Geometry: final body of the model. Coordinates: model frame, mm. A direction names the side the tool comes from. Round coordinates to 2 decimals unless told otherwise and drop trailing zeros. Write each loop counter-clockwise with the first axis right and the second up, starting at its lowest first coordinate (ties: lowest second). Pieces come first, ordered by that corner, then holes. Notation, with made-up numbers: (29, -38) -> (38, -38) arc R25 cw to (38, -14) -> close; hole circle Ø8 at (17.25, 13). An arc over 180 degrees is marked (long way). One line per item, written item: value. Start each with the question number.
from build123d import *

# Parameters (mm, degrees)
BOSS_EXTRUDE1_DEPTH            = 6.4
SKETCH2_R                      = 6.92820323
BOSS_EXTRUDE2_DEPTH            = 9.2
SKETCH3_R                      = 1.65
CUT_EXTRUDE3_DEPTH             = 16.6
SKETCH4_W                      = 5.65
SKETCH4_H                      = 2.55
CUT_EXTRUDE4_DEPTH             = 6.4
CUT_EXTRUDE5_REACH             = 4.978
SKETCH5_R                      = 1.5
CUT_EXTRUDE5_DIRECTION_2_REACH = 12.878
CUT_EXTRUDE7_DEPTH             = 2.55
SKETCH3_4_R                    = 2.05
SKETCH3_4_R_2                  = 1.65
CUT_EXTRUDE8_DEPTH             = 9.4
CHAMFER1_SIZE                  = 0.3


with BuildPart() as part:
    # Sketch1 → Boss-Extrude1 (new body)
    with BuildSketch(Plane(origin=(0, 0, 0), x_dir=(1, 0, 0), z_dir=(0, 1, 0))):
        Polygon((3.170646703, -6.160113594), (6.920138214, -0.334196206), (3.749491511, 5.825917388), (-3.170646703, 6.160113594), (-6.920138214, 0.334196206), (-3.749491511, -5.825917388), align=None)
    extrude(amount=BOSS_EXTRUDE1_DEPTH)

    # Sketch2 → Boss-Extrude2 (add)
    with BuildSketch(Plane(origin=(0, 6.4, 0), x_dir=(1, 0, 0), z_dir=(0, 1, 0))):
        Circle(SKETCH2_R)
    extrude(amount=BOSS_EXTRUDE2_DEPTH)

    # Sketch3 → Cut-Extrude3 (cut, through all)
    with BuildSketch(Plane(origin=(0, 15.6, 0), x_dir=(1, 0, 0), z_dir=(0, 1, 0))):
        Circle(SKETCH3_R)
    extrude(amount=-CUT_EXTRUDE3_DEPTH, mode=Mode.SUBTRACT)

    # Sketch4 → Cut-Extrude4 (cut)
    with BuildSketch(Plane(origin=(0, 15.6, 0), x_dir=(1, 0, 0), z_dir=(0, 1, 0))):
        with Locations((0, 2.675)):
            Rectangle(SKETCH4_W, SKETCH4_H)
    extrude(amount=-CUT_EXTRUDE4_DEPTH, mode=Mode.SUBTRACT)

    # Sketch5 → Cut-Extrude5 (cut, up to next)
    with BuildSketch(Plane.XY.offset(-3.95), mode=Mode.PRIVATE) as cut_extrude5_sk1:
        with Locations((0, 10.8)):
            Circle(SKETCH5_R)
    cut_extrude5_tool1 = extrude(cut_extrude5_sk1.sketch, amount=-CUT_EXTRUDE5_REACH, mode=Mode.PRIVATE) & part.part
    add(cut_extrude5_tool1.solids().sort_by_distance((0, 10.8, -3.95))[0], mode=Mode.SUBTRACT)

    # Sketch5 → Cut-Extrude5 direction 2 (cut, up to next)
    with BuildSketch(Plane.XY.offset(-3.95), mode=Mode.PRIVATE) as cut_extrude5_direction_2_sk1:
        with Locations((0, 10.8)):
            Circle(SKETCH5_R)
    cut_extrude5_direction_2_tool1 = extrude(cut_extrude5_direction_2_sk1.sketch, amount=CUT_EXTRUDE5_DIRECTION_2_REACH, mode=Mode.PRIVATE) & part.part
    add(cut_extrude5_direction_2_tool1.solids().sort_by_distance((0, 10.8, -3.95))[0], mode=Mode.SUBTRACT)

    # Sketch7 → Cut-Extrude7 (cut)
    with BuildSketch(Plane.XY.offset(-3.95)):
        Polygon((-2.825, 12.437789047), (-2.830866921, 9.172372758), (-0.005866921, 7.534583711), (2.825, 9.162210953), (2.830866921, 12.427627242), (0.005866921, 14.065416289), align=None)
    extrude(amount=CUT_EXTRUDE7_DEPTH, mode=Mode.SUBTRACT)

    # Sketch3_4 → Cut-Extrude8 (cut)
    with BuildSketch(Plane(origin=(0, 15.6, 0), x_dir=(1, 0, 0), z_dir=(0, 1, 0))):
        Circle(SKETCH3_4_R)
        Circle(SKETCH3_4_R_2, mode=Mode.SUBTRACT)
    extrude(amount=-CUT_EXTRUDE8_DEPTH, mode=Mode.SUBTRACT)

    # Chamfer1
    chamfer1_edges = [part.edges().sort_by_distance(p)[0] for p in [
        (-1.65, 0, 0),
        (-5.334814862, 0, 2.745860591),
        (-5.045392458, 0, -3.2471549),
        (0.289422404, 0, -5.993015491),
        (5.334814862, 0, -2.745860591),
        (5.045392458, 0, 3.2471549),
        (-0.289422404, 0, 5.993015491),
    ]]
    chamfer(chamfer1_edges, length=CHAMFER1_SIZE)


solid = part.part
(1) Set-up query: faces 5 (the face through (-5.3, 6.4, -3.5)), 6 (the face through (-1.438, 8.365, -2.693)), 7 (the face through (5.3, 6.4, 3.4)), 8 (the face through (-0.3, 6.4, 6.4)), 9 (the face through (0.34, 3.31, -5.99)). Return all of +Z, -Z, +X, -X, +Y, -Y with unobstructed straight access to the full face (end or side cutting, diameter ignored); none if empty.
(2) Line query: probe 1 along Y at (x, z) = (-5.25, 3); probe 2 along Y at (x, z) = (0, -4.55); probe 3 along X at (y, z) = (10.8, -6.25). Output: solid intervals per line, ascending.
(3) Pin query (flat end, axial travel): pin 1 (3.5 mm diameter, centred on x = 0, z = 0, fed in from -Y); pin 2 (3.5 mm diameter, centred on x = 0, z = 0, fed in from +Y); pin 3 (4 mm diameter, centred on x = 4.5, y = 4.5, fed in from +Z). Return the tip coordinate at first contact, or that it passes through.
(4) Section query D-D (x = -0.5). Count the separate pieces of the cut face and the enclosed holes in it, and give its area (3 significant figures).
(5) Section query A-A (y = 4.25). Output: boundary loops of the cut face in (x, z).
(6) Pull-direction query (X, two-part tool) for faces 1 (the face through (-6, 6.4, 3)), 2 (the face through (-5.36, 3.31, 2.7)), 3 (the face through (-0.325, 9.336, -5.421)), 4 (the face through (-1.216, 3.291, -1.115)); classes: pulls with the +X half, pulls with the -X half, needs draft (parallel to the pull), parting line crosses it, or undercut.
(7) Section query B-B (x = 2.5). Output: boundary loops of the cut face in (y, z), and give its area (3 significant figures).
(8) Section query C-C (z = 0). Output: boundary loops of the cut face in (x, y), and give its area (3 significant figures).
Results list:
1. face 5: -Z, -X, -Y
1. face 6: +Y
1. face 7: +Z, +X, -Y
1. face 8: +Z, -X, -Y
1. face 9: -Z, +X, -Y
2. probe 1: y = 6.4 to 15.6
2. probe 2: y = 0 to 9.3, 12.3 to 15.6
2. probe 3: x = -2.99 to -1.5, 1.5 to 2.99
3. pin 1: stops at y = 0.2
3. pin 2: stops at y = 6.2
3. pin 3: stops at z = 6.16
4. separate pieces: 3
4. enclosed holes: 0
4. area: 123 mm^2
5. outline: (-6.92, -0.33) -> (-3.17, -6.16) -> (3.75, -5.83) -> (6.92, 0.33) -> (3.17, 6.16) -> (-3.75, 5.83) -> close; hole circle Ø3.3 at (0, 0)
6. face 1: needs draft
6. face 2: pulls with the -X half
6. face 3: undercut
6. face 4: undercut
7. outline: (0, -5.59) -> (0.3, -5.89) -> (6.4, -5.89) -> (6.4, -6.46) -> (15.6, -6.46) -> (15.6, -3.95) -> (8.98, -3.95) -> (8.98, -1.4) -> (15.6, -1.4) -> (15.6, 6.46) -> (6.4, 6.46) -> (6.4, 6.13) -> (0.3, 6.13) -> (0, 5.83) -> close
7. area: 179 mm^2
8. outline: (-6.93, 6.4) -> (-6.75, 6.4) -> (-6.75, 0.3) -> (-6.41, 0) -> (-1.95, 0) -> (-1.65, 0.3) -> (-1.65, 6.2) -> (-2.05, 6.2) -> (-2.05, 15.6) -> (-6.93, 15.6) -> close; (1.65, 0.3) -> (1.95, 0) -> (6.41, 0) -> (6.75, 0.3) -> (6.75, 6.4) -> (6.93, 6.4) -> (6.93, 15.6) -> (2.05, 15.6) -> (2.05, 6.2) -> (1.65, 6.2) -> close
8. area: 155 mm^2
